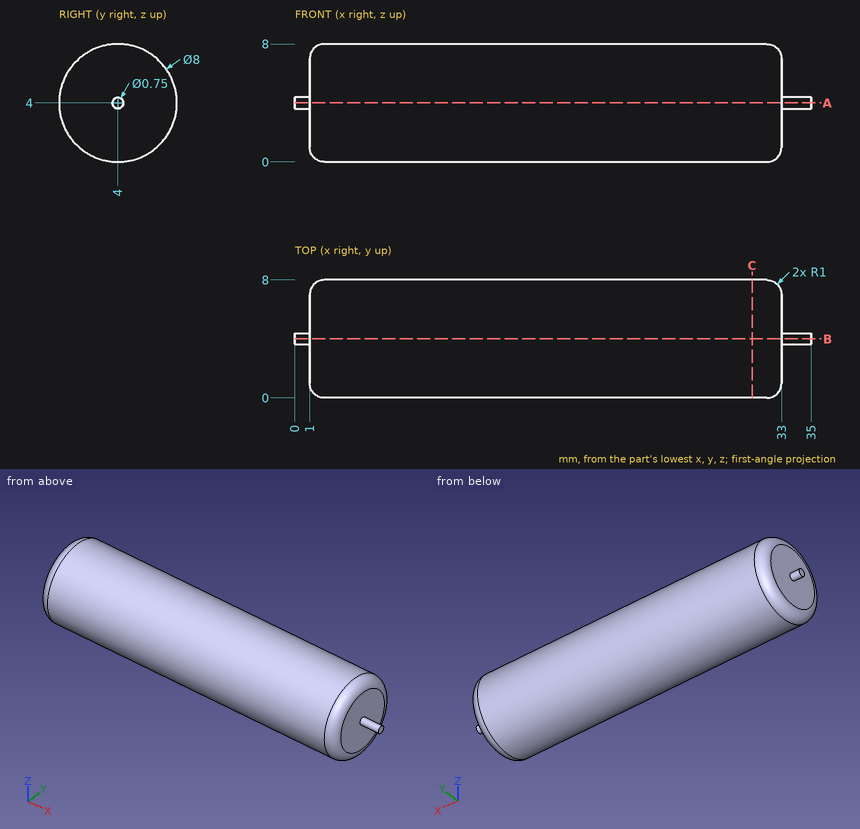
The drawing under review shows one solid part. Ordinate dimensions are in mm from its lowest x, y, z. Round coordinates to 2 decimals unless told otherwise and drop trailing zeros. Loops run counter-clockwise (first coordinate to the right, second up) from the corner with the lowest first, then second, coordinate; pieces in that order, holes last. Notation, with made-up numbers: M 46,20 L 86,20 A37 ccw 86,58 Z; hole C -12,1.5 d5. An arc over 180 degrees is marked long. Answer as CSV lines item,"result". Start each with the question number.
Item 1: Insertion check: P1, Ø3, axis at x = 28, y = 2, coming from the -Z side; P2, Ø2, axis at x = 9, y = 7, coming from the -Z side; P3, Ø4, axis at y = 2, z = 6, coming from the -X side. Each pin has a flat end and moves straight along its axis. Give the tip position at first contact, or say it passes through.
Item 2: Consider section A-A (z = 4). Write out the cut boundary in (x, y) (3 decimals), then the cut area to 3 significant figures.
Item 3: Consider section C-C (x = 31). Write out the cut boundary in (y, z), then the cut area to 3 significant figures.
Item 4: Wall thickness on line 1 (X direction, y = 1.5, z = 4.5); line 2 (Y direction, x = 28.5, z = 2.25); line 3 (Z direction, x = 10, y = 3.5): over which ranges is each line inside the solid? List them lowest first. Write a range as [from, to].
Answer:
1,P1,"stops at z = 0.03"
1,P2,"stops at z = 0.54"
1,P3,"stops at x = 1"
2,outline,"M 0,3.625 L 1,3.625 L 1,1 A1 ccw 2,0 L 32,0 A1 ccw 33,1 L 33,3.625 L 35,3.625 L 35,4.375 L 33,4.375 L 33,7 A1 ccw 32,8 L 2,8 A1 ccw 1,7 L 1,4.375 L 0,4.375 Z"
2,area,"257 mm^2"
3,outline,"C 4,4 d8"
3,area,"50.3 mm^2"
4,line 1,"x = [1, 33]"
4,line 2,"y = [0.4, 7.6]"
4,line 3,"z = [0.03, 7.97]"
